from build123d import *

# Parameters (mm, degrees)
SKICA1_W                = 77
SKICA1_H                = 21
P_IDAT_VYSUNUT_M1_DEPTH = 19.5
ZAOBLIT1_R              = 8


with BuildPart() as part:
    # Skica1 → Přidat vysunutím1 (new body)
    with BuildSketch(Plane.XY):
        Rectangle(SKICA1_W, SKICA1_H)
    extrude(amount=P_IDAT_VYSUNUT_M1_DEPTH)

    # Zaoblit1
    zaoblit1_edges = [part.edges().sort_by_distance(p)[0] for p in [
        (0, -10.5, 19.5),
        (0, 10.5, 19.5),
    ]]
    fillet(zaoblit1_edges, radius=ZAOBLIT1_R)


solid = part.part
Geometry: final body of the model. Coordinates: model frame, mm. Give positions to 0.01 mm unless a question says otherwise; leave off trailing zeros. Write each loop counter-clockwise with the first axis right and the second up, starting at its lowest first coordinate (ties: lowest second). Pieces come first, ordered by that corner, then holes. Notation, with made-up numbers: (23.5, -31) -> (63.5, -31) arc R26 ccw to (63.5, -16) -> close; hole circle Ø10 at (60, -33.75). An arc over 180 degrees is marked (long way). Answer as a JSON object with one key per item and string values.
1. Contact query for a flat-ended pin moving along its axis: pin 1 (4 mm diameter, centred on x = -0.5, y = 7.5, fed in from +Z). Output: stop coordinate, or through.
Ans:
{"pin 1": "stops at z = 18.92"}
2. Ray query, probe 1 along Z at (x, y) = (-28, 3); probe 2 along Y at (x, z) = (-9, 12); probe 3 along Z at (x, y) = (6, 9.75). Return the intervals inside material, ascending. Write a range as from..to.
Ans:
{"probe 1": "z = 0..19.48", "probe 2": "y = -10.48..10.48", "probe 3": "z = 0..14.88"}
3. Cut plane C-C on z = 14.75. Output: boundary loops of the cut face in (x, y).
Ans:
{"outline": "(-38.5, -9.81) -> (38.5, -9.81) -> (38.5, 9.81) -> (-38.5, 9.81) -> close"}
4. Cut plane A-A on x = -22.5. Output: boundary loops of the cut face in (y, z).
Ans:
{"outline": "(-10.5, 0) -> (10.5, 0) -> (10.5, 11.5) arc R8 ccw to (2.5, 19.5) -> (-2.5, 19.5) arc R8 ccw to (-10.5, 11.5) -> close"}
5. Cut plane B-B on y = -9. Output: boundary loops of the cut face in (x, z).
Ans:
{"outline": "(-38.5, 0) -> (38.5, 0) -> (38.5, 16.16) -> (-38.5, 16.16) -> close"}
